```python
from build123d import *

# Parameters (mm, degrees)
F2_R     = 55
F3_DEPTH = 245
F4_R     = 92.5
F4_R_2   = 55
F5_DEPTH = 10


with BuildPart() as f1:
    # F0 (on Front) → F1 (revolve)
    with BuildSketch(Plane.XZ):
        with BuildLine():
            Line((0, 155), (0, 0))
            Line((0, 0), (207, 0))
            Line((207, 0), (207, 7))
            Line((207, 7), (214, 7))
            Line((214, 7), (214, 45))
            ThreePointArc((214, 45), (216.928932, 52.071068), (224, 55))
            Line((224, 55), (254, 55))
            Line((254, 55), (254, 100))
            Line((254, 100), (224, 100))
            ThreePointArc((224, 100), (216.928932, 102.928932), (214, 110))
            Line((214, 110), (214, 148))
            Line((214, 148), (207, 148))
            Line((207, 148), (207, 155))
            Line((207, 155), (0, 155))
        make_face()
    revolve(axis=Axis((0, 0, 77.5), (0, 0, 1)))

    # F2 (on Front) → F3 (join)
    with BuildSketch(Plane.XZ):
        with Locations((167, 77.5)):
            Circle(F2_R)
    extrude(amount=F3_DEPTH)

    # F4 (on face) → F5 (join)
    with BuildSketch(Plane.XZ.offset(245)):
        with Locations((167, 77.5)):
            Circle(F4_R)
        with Locations((167, 77.5)):
            Circle(F4_R_2, mode=Mode.SUBTRACT)
        with Locations((167, 77.5)):
            Circle(F4_R_2)
    extrude(amount=F5_DEPTH)


solid = f1.part
```
Build history of the part. All positions in model axes, mm. A direction names the side the tool comes from. Give positions to 0.01 mm unless a question says otherwise; leave off trailing zeros. Order: outer loops, then holes, each group sorted by start corner. A loop starts at its lowest first (then second) coordinate and runs counter-clockwise, first axis right, second up. Notation, with made-up numbers: M 49.5,-6.5 L 108.5,-6.5 A26 ccw 108.5,16.5 Z; hole C -20,-31 d4. An arc over 180 degrees is marked long. Return JSON: item names as keys, results as strings.
Q1. Band-saw the part on A-A (y = 0). Give the cut face in (x, z), then the cut area to 3 significant figures.
Answer list:
{"outline": "M -254,55 L -224,55 A10 cw -214,45 L -214,7 L -207,7 L -207,0 L 207,0 L 207,7 L 214,7 L 214,45 A10 cw 224,55 L 254,55 L 254,100 L 224,100 A10 cw 214,110 L 214,148 L 207,148 L 207,155 L -207,155 L -207,148 L -214,148 L -214,110 A10 cw -224,100 L -254,100 Z", "area": "69,800 mm^2"}
Q2. Wall check: probe 1 along Z at (x, y) = (-28, -47.5); probe 2 along Z at (x, y) = (-164, -127); probe 3 along Y at (x, z) = (222, 149). Give the ranges that are in metal, low to high. Write a range as from..to.
Answer list:
{"probe 1": "z = 0..155", "probe 2": "z = 7..148", "probe 3": "y = -255..-245"}
Q3. Band-saw the part on C-C (z = 64). Give the cut face in (x, y).
Answer list:
{"outline": "M 75.49,-255 L 258.51,-255 L 258.51,-245 L 220.32,-245 L 220.32,-126.4 A254 ccw long 113.68,-227.14 L 113.68,-245 L 75.49,-245 Z"}
Q4. Band-saw the part on D-D (z = 142). Give the cut face in (x, y), then the cut area to 3 significant figures.
Answer list:
{"outline": "C 0,0 d428; M 100.7,-255 L 233.3,-255 L 233.3,-245 L 100.7,-245 Z", "area": "145,000 mm^2"}
Q5. 3-axis set-ups, long thin cutter, end or side, ignore diameter. For faces 1 (the face through (-3, 3, 155)), 2 (the face through (-149, 171, 55)), 3 (the face through (207, -245, 38)): which of +Z, -Z, +X, -X, +Y, -Y reach the whole face in a straight line?
Answer list:
{"face 1": "+Z, +X, -X, +Y", "face 2": "-Z", "face 3": "none"}
Q6. Flat gauge pins, fed straight in: pin 1 (10 mm diameter, centred on x = -64.5, y = -40, fed in from -Z); pin 2 (1.5 mm diameter, centred on x = -113.5, y = -24.5, fed in from +Z); pin 3 (1 mm diameter, centred on x = -145, z = 37.5, fed in from +Y). Where does each tip first touch, or does it go through?
Answer list:
{"pin 1": "stops at z = 0", "pin 2": "stops at z = 155", "pin 3": "stops at y = 157.85"}
Q7. Two-plate mould, pull along Y, no slides. Class faces 4 (the face through (166, -255, 79)), 5 (the face through (255.23, -249.93, 105.28)), 6 (the face through (-112, 175, 148)): pulls with the +Y half, pulls with the -Y half, needs draft (parallel to the pull), parting line crosses it, or undercut.
Answer list:
{"face 4": "pulls with the -Y half", "face 5": "needs draft", "face 6": "undercut"}
